Could you check a few things on this drawing? It's one solid part, dimensions in mm from its lowest x, y, z. Coordinates: 2 decimals unless noted, no trailing zeros. Order: outer loops, then holes, each group sorted by start corner. A loop starts at its lowest first (then second) coordinate and runs counter-clockwise, first axis right, second up.
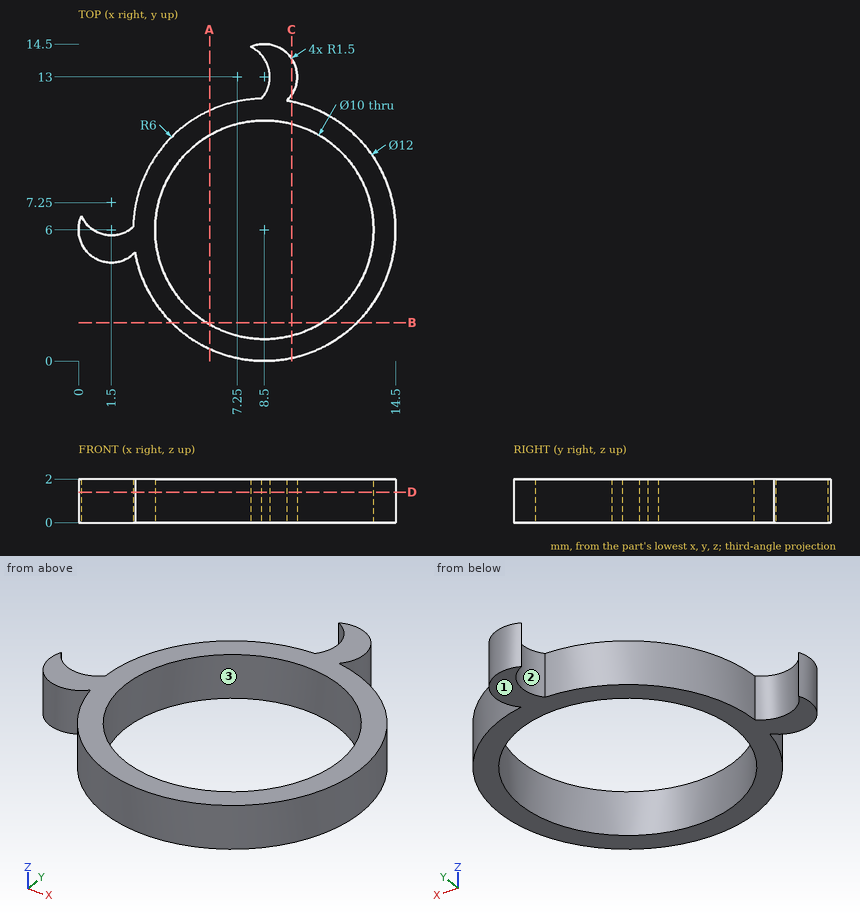
1. Thinking about a two-plate mould opening in X: for the marked faces 1, 2 and 3, which applies, pulls with the +X half, pulls with the -X half, needs draft (parallel to the pull), parting line crosses it, or undercut?
Completed:
face 1: needs draft
face 2: pulls with the -X half
face 3: undercut
2. Imagine slicing it at D-D on z = 1.4. Please give me the cut outline in (x, y) (3 decimals), then the cut area to 3 significant figures.
Completed:
outline: (0.136, 6.625) arc R1.5 ccw to (2.589, 4.969) arc R6 ccw (long way) to (9.531, 11.911) arc R1.5 ccw to (7.875, 14.364) arc R1.5 cw to (8.367, 11.999) arc R6 ccw to (2.501, 6.133) arc R1.5 cw to start; hole circle Ø10 at (8.5, 6)
area: 40.8 mm2
3. I'm going to push flat-ended pins straight in: pin 1 (8 mm diameter, centred on x = 8, y = 2.5, fed in from -Z); pin 2 (1 mm diameter, centred on x = 12, z = 1.5, fed in from -Y). Where does each tip first touch, or does it pass through?
Completed:
pin 1: stops at z = 0
pin 2: stops at y = 0.8
4. Imagine slicing it at C-C on x = 9.75. Please give me the cut outline in (y, z).
Completed:
outline: (0.13, 0) - (1.16, 0) - (1.16, 2) - (0.13, 2) - close; (10.84, 0) - (11.87, 0) - (11.87, 2) - (10.84, 2) - close; (12.17, 0) - (13.83, 0) - (13.83, 2) - (12.17, 2) - close
5. Imagine slicing it at B-B on y = 1.75. Please give me the cut outline in (x, z), then the cut area to 3 significant figures.
Completed:
outline: (4.26, 0) - (5.87, 0) - (5.87, 2) - (4.26, 2) - close; (11.13, 0) - (12.74, 0) - (12.74, 2) - (11.13, 2) - close
area: 6.41 mm2
6. Imagine slicing it at A-A on x = 6. Please give me the cut outline in (y, z), then the cut area to 3 significant figures.
Completed:
outline: (0.55, 0) - (1.67, 0) - (1.67, 2) - (0.55, 2) - close; (10.33, 0) - (11.45, 0) - (11.45, 2) - (10.33, 2) - close
area: 4.50 mm2
7. Please list where these lines run through material, in increasing order: probe 1 along Y at (x, z) = (8.5, 0.9); probe 2 along Y at (x, z) = (12.25, 1.2); probe 3 along Y at (x, z) = (9.5, 1.55).
Completed:
probe 1: y = 0 to 1, 11 to 12.17, 13.83 to 14.5
probe 2: y = 1.32 to 2.69, 9.31 to 10.68
probe 3: y = 0.08 to 1.1, 10.9 to 14.12
